Build history of the part. All positions in model axes, mm. A direction names the side the tool comes from. Coordinates: 2 decimals unless noted, no trailing zeros. Loops run counter-clockwise (first coordinate to the right, second up) from the corner with the lowest first, then second, coordinate; pieces in that order, holes last.
(1) Two-plate mould, pull along X, no slides. Class faces 4 (the face through (164.76, -8.85, 0.84)), 5 (the face through (10, 50, 0)), 6 (the face through (-34.584, 24.739, 0.35)): pulls with the +X half, pulls with the -X half, needs draft (parallel to the pull), parting line crosses it, or undercut.
(2) Slice it at C-C (y = -12.5). Give the number of separate pieces and of enclosed holes in the cut face, and give its area (3 significant figures).
(3) Wall check: L1, parallel to X at y = -12.5, z = 10; L2, parallel to X at y = -16, z = -37.5; L3, parallel to X at y = -14, z = -40. Give the ranges that are in metal, low to high.
(4) Tool access for faces 1 (the face through (1, 25, 25)), 2 (the face through (21.8, 25.37, 2.25)), 3 (the face through (50.56, -8.85, -44.76)): list every direction of +Z, -Z, +X, -X, +Y, -Y with a clear straight run to the whole face (end or side of a thin tool).
(5) Flat gauge pins, fed straight in: P1, Ø20, axis at x = 1, y = -6.5, coming from the -Z side; P2, Ø12, axis at x = 138.5, y = 1, coming from the +Z side; P3, Ø8, axis at y = 23.5, z = 15, coming from the -X side; P4, Ø8, axis at x = 89.5, y = -7, coming from the +Z side. Where does each tip first touch, or does it go through?
(6) Slice it at A-A (x = 11.5). Give the cut face in (y, z).
(7) Slice it at B-B (z = 10). Give the cut face in (x, y), and give its area (3 significant figures).
(8) Slice it at D-D (y = 2.5). Give the cut face in (x, z).
from build123d import *

# Parameters (mm, degrees)
EXTRUDE_3_DEPTH     = 40
FILLET_1_R          = 20
SKETCH_17_R         = 10
CUT_EXTRUDE_2_DEPTH = 88.749643874
CHAMFER_1_SIZE      = 20
CHAMFER_1_SIZE2     = 34.641016151
SWEEP_2_PROFILE_R   = 7.5
SWEEP_2_2_PROFILE_R = 6


with BuildPart() as part:
    # 草图15 → 凸台-拉伸3 (new, symmetric)
    with BuildSketch(Plane(origin=(0, 0, 0), x_dir=(0, 0, -1), z_dir=(1, 0, 0))):
        Polygon((-60, 0), (-25, 0), (-25, 50), (25, 50), (25, 0), (60, 0), (60, -25), (-60, -25), align=None)
    extrude(amount=EXTRUDE_3_DEPTH, both=True)

    # 圆角1
    fillet_1_edges = [part.edges().sort_by_distance(p)[0] for p in [
        (-40, -12.5, -60),
        (-40, -12.5, 60),
    ]]
    fillet(fillet_1_edges, radius=FILLET_1_R)

    # 草图17 → 切除-拉伸2 (cut, through all)
    with BuildSketch(Plane(origin=(0, 0, 0), x_dir=(1, 0, 0), z_dir=(0, 1, 0))):
        with Locations(Location((-20, 40, 0), (0, 0, 270))):
            Circle(SKETCH_17_R)
    cut_extrude_2 = extrude(amount=-CUT_EXTRUDE_2_DEPTH, mode=Mode.SUBTRACT)

    # 镜向1: 切除-拉伸2 across plane
    add(cut_extrude_2.mirror(Plane.XY), mode=Mode.SUBTRACT)

    # 倒角1
    chamfer_1_edges = [part.edges().sort_by_distance(p)[0] for p in [
        (-40, 50, 0),
    ]]
    chamfer_1_side = [part.faces().sort_by_distance(p)[0] for p in [
        (0, 50, 0),
    ]]
    chamfer(chamfer_1_edges, length=CHAMFER_1_SIZE, length2=CHAMFER_1_SIZE2, reference=chamfer_1_side[0])

    # Sweep 2: sweep along a path in 草图19
    with BuildLine(Plane.XY) as sweep_2_path:
        Line((-30, 32.679491924), (-11.908563538, 22.234396213))
        ThreePointArc((-11.908563538, 22.234396213), (-4.673134891, 19.237383538), (3.091436462, 18.215158327))
        Line((3.091436462, 18.215158327), (40, 18.215158327))
    # Sweep 2 profile (on start of the path) → Sweep 2 (sweep, cut)
    with BuildSketch(Plane(origin=(-30, 32.679491924, 0), x_dir=(0.500000000000001, 0.866025403784438, 0), z_dir=(0.866025403784438, -0.500000000000001, 0))):
        Circle(SWEEP_2_PROFILE_R)
    sweep(path=sweep_2_path.line, mode=Mode.SUBTRACT)

    # Sweep 2 2: sweep along a path in 草图26
    with BuildLine(Plane(origin=(0, -12.5, 0), x_dir=(1, 0, 0), z_dir=(0, 1, 0))) as sweep_2_2_path:
        Line((40, 40), (60.827915323, 40))
        ThreePointArc((60.827915323, 40), (69.165079187, 41.820569352), (75.984404551, 46.95083013))
        Line((75.984404551, 46.95083013), (98.454098123, 73.04916987))
        ThreePointArc((98.454098123, 73.04916987), (105.273423486, 78.179430648), (113.610587351, 80))
        Line((113.610587351, 80), (140, 80))
        ThreePointArc((140, 80), (154.142135624, 74.142135624), (160, 60))
        Line((160, 60), (160, -60))
        ThreePointArc((160, -60), (154.142135624, -74.142135624), (140, -80))
        Line((140, -80), (113.610587351, -80))
        ThreePointArc((113.610587351, -80), (105.273423486, -78.179430648), (98.454098123, -73.04916987))
        Line((98.454098123, -73.04916987), (75.984404551, -46.95083013))
        ThreePointArc((75.984404551, -46.95083013), (69.165079187, -41.820569352), (60.827915323, -40))
        Line((60.827915323, -40), (40, -40))
    # Sweep 2 2 profile (on start of the path) → Sweep 2 2 (sweep)
    with BuildSketch(Plane(origin=(40, -12.5, -40), x_dir=(0, 0, 1), z_dir=(1, 0, 0))):
        Circle(SWEEP_2_2_PROFILE_R)
    sweep(path=sweep_2_2_path.line)


solid = part.part
Response values:
1. face 4: undercut
1. face 5: needs draft
1. face 6: pulls with the -X half
2. separate pieces: 1
2. enclosed holes: 3
2. area: 13,800 mm2
3. L1: x = -40 to 40, 154 to 166
3. L2: x = -40 to -29.68, -10.32 to 71.43, 155.13 to 164.87
3. L3: x = -40 to -30, -10 to 77.14, 154.19 to 165.81
4. face 1: +Z, +X, -X, +Y
4. face 2: +X
4. face 3: none
5. P1: stops at z = -60
5. P2: passes through
5. P3: stops at x = -37.61
5. P4: stops at z = 74.24
6. outline: (-25, -60) - (0, -60) - (0, -25) - (50, -25) - (50, 25) - (0, 25) - (0, 60) - (-25, 60) - close; hole circle Ø15 at (18.22, 0)
7. outline: (-40, -25) - (40, -25) - (40, 50) - (-20, 50) - (-40, 15.36) - close; circle Ø12 at (160, -12.5)
7. area: 5,770 mm2
8. outline: (-40, -25) - (40, -25) - (40, 25) - (-40, 25) - close
